Part model, mm, in its own coordinate system. A direction names the side the tool comes from. Give positions to 0.01 mm unless a question says otherwise; leave off trailing zeros. Write each loop counter-clockwise with the first axis right and the second up, starting at its lowest first coordinate (ties: lowest second). Pieces come first, ordered by that corner, then holes.
from build123d import *

# Parameters (mm, degrees)
F0_R     = 2.4
F1_DEPTH = 7
F2_W     = 85
F2_H     = 17
F3_DEPTH = 1
F4_R     = 5
F5_R     = 2
F6_SIZE  = 1.8


with BuildPart() as f1:
    # F0 (on Front) → F1 (new body)
    with BuildSketch(Plane.XZ):
        Polygon((42.5, -23.5), (42.5, 23.5), (-42.5, 23.5), (-42.5, -23.5), (-20, -23.5), align=None)
        with BuildLine():
            ThreePointArc((-17.6, 2.5), (-18.3029437252, 0.8029437252), (-20, 0.1))
            ThreePointArc((-20, 0.1), (-21.6970562748, 4.1970562748), (-17.6, 2.5))
        make_face(mode=Mode.SUBTRACT)
        with Locations((-30, 16.5)):
            Circle(F0_R, mode=Mode.SUBTRACT)
        with Locations((20, 2.5)):
            Circle(F0_R, mode=Mode.SUBTRACT)
        with Locations((30, 16.5)):
            Circle(F0_R, mode=Mode.SUBTRACT)
    extrude(amount=F1_DEPTH)

    # F2 (on face) → F3 (join)
    with BuildSketch(Plane(origin=(0, 0, 0), x_dir=(-1, 0, 0), z_dir=(0, 1, 0))):
        with Locations((0, -15)):
            Rectangle(F2_W, F2_H)
    extrude(amount=F3_DEPTH)

    # F4
    f4_edges = [f1.edges().sort_by_distance(p)[0] for p in [
        (42.5, -3.5, 23.5),
        (-42.5, -3.5, 23.5),
        (42.5, -3, -23.5),
        (-42.5, -3, -23.5),
    ]]
    fillet(f4_edges, radius=F4_R)

    # F5
    f5_edges = [f1.edges().sort_by_distance(p)[0] for p in [
        (0, -7, -23.5),
    ]]
    fillet(f5_edges, radius=F5_R)

    # F6
    f6_edges = [f1.edges().sort_by_distance(p)[0] for p in [
        (17.6, -7, 2.5),
        (27.6, -7, 16.5),
        (-22.4, -7, 2.5),
        (-32.4, -7, 16.5),
    ]]
    chamfer(f6_edges, length=F6_SIZE)


solid = f1.part
1) 3-axis set-ups, long thin cutter, end or side, ignore diameter. For faces 1 (the flat face through (-42.5, -2, 0)), 2 (the flat face through (-1, 0, 9)): which of +Z, -Z, +X, -X, +Y, -Y reach the whole face in a straight line?
Check result:
face 1: +Z, -Z, -X, +Y, -Y
face 2: +Z, +X, -X, +Y
2) Saw through at D-D (x = -36). Write the cut outline in (y, z).
Check result:
outline: (-7, -21.5) arc R2 ccw to (-5, -23.5) - (1, -23.5) - (1, -6.5) - (0, -6.5) - (0, 23.5) - (-5, 23.5) arc R2 ccw to (-7, 21.5) - close
3) Saw through at A-A (x = 30). Write the cut outline in (y, z), and give its area (3 significant figures).
Check result:
outline: (-7, -21.5) arc R2 ccw to (-5, -23.5) - (1, -23.5) - (1, -6.5) - (0, -6.5) - (0, 14.1) - (-5.2, 14.1) - (-7, 12.3) - close; (-7, 20.7) - (-5.2, 18.9) - (0, 18.9) - (0, 23.5) - (-5, 23.5) arc R2 ccw to (-7, 21.5) - close
area: 307 mm2
4) Flat gauge pin, fed straight in: P1, Ø5, axis at x = -18.5, z = 17, coming from the +Y side. Where does the tip first touch, or does it go through?
Check result:
P1: stops at y = 0
5) Mould opens along X. For faces 3 (the cylindrical face through (-41, -1.96, -22.07)), 4 (the flat face through (1, -2, 23.5)), 5 (the cylindrical face through (32.217, -2.564, 15.581)) say: +X half, -X half, draft (parallel to the pull), parting line (faces both ways), or undercut.
Check result:
face 3: -X half
face 4: draft
face 5: undercut
6) Saw through at B-B (z = 16.5). Write the cut outline in (x, y).
Check result:
outline: (-42.5, -5) arc R2 ccw to (-40.5, -7) - (-34.2, -7) - (-32.4, -5.2) - (-32.4, 0) - (-42.5, 0) - close; (-27.6, -5.2) - (-25.8, -7) - (25.8, -7) - (27.6, -5.2) - (27.6, 0) - (-27.6, 0) - close; (32.4, -5.2) - (34.2, -7) - (40.5, -7) arc R2 ccw to (42.5, -5) - (42.5, 0) - (32.4, 0) - close
7) Saw through at C-C (y = -2). Write the cut outline in (x, z).
Check result:
outline: (-42.5, -18.5) arc R5 ccw to (-37.5, -23.5) - (37.5, -23.5) arc R5 ccw to (42.5, -18.5) - (42.5, 18.5) arc R5 ccw to (37.5, 23.5) - (-37.5, 23.5) arc R5 ccw to (-42.5, 18.5) - close; hole circle Ø4.8 at (-30, 16.5); hole circle Ø4.8 at (-20, 2.5); hole circle Ø4.8 at (20, 2.5); hole circle Ø4.8 at (30, 16.5)
8) Drill centre lines: L1, parallel to Z at x = 20, y = -2; L2, parallel to Z at x = -30, y = -3.8; L3, parallel to Y at x = -22, z = 16. Where is each one in solid material? Low to high.
Check result:
L1: z = -23.5 to 0.1, 4.9 to 23.5
L2: z = -23.5 to 14.1, 18.9 to 23.5
L3: y = -7 to 0
